Can you work these out from the model? Positions are in its coordinate system, mm. A direction names the side the tool comes from. Coordinates: 2 decimals unless noted, no trailing zeros. Order: outer loops, then holes, each group sorted by start corner. A loop starts at its lowest first (then second) coordinate and runs counter-clockwise, first axis right, second up.
```python
from build123d import *

# Parameters (mm, degrees)
F0_R     = 10
F1_DEPTH = 12


with BuildPart() as f1:
    # F0 (on Front) → F1 (new body)
    with BuildSketch(Plane.XZ):
        with BuildLine():
            Line((0, 20), (0, 0))
            Line((0, 0), (20, 0))
            Line((20, 0), (20, -10))
            Line((20, -10), (84, -10))
            Line((84, -10), (84, 0))
            Line((84, 0), (104, 0))
            Line((104, 0), (104, 20))
            ThreePointArc((104, 20), (92.284271, 48.284271), (64, 60))
            Line((64, 60), (40, 60))
            ThreePointArc((40, 60), (11.715729, 48.284271), (0, 20))
        make_face()
        with Locations((52, 40)):
            Circle(F0_R, mode=Mode.SUBTRACT)
    extrude(amount=F1_DEPTH)


solid = f1.part
```
1. Please list where these lines run through material, in increasing order: probe 1 along Z at (x, y) = (52, -3.25); probe 2 along Z at (x, y) = (59, -5); probe 3 along Z at (x, y) = (72, -9.5).
Completed:
probe 1: z = -10 to 30, 50 to 60
probe 2: z = -10 to 32.86, 47.14 to 60
probe 3: z = -10 to 59.19
2. Thinking about a two-plate mould opening in X: for faces 1 (the cylindrical face through (92.594, -5.916, 47.972)), 2 (the cylindrical face through (44, -6, 34)), 3 (the cylindrical face through (12.028, -5.916, 48.594)), 4 (the flat face through (51, -12, 25)), which applies, pulls with the +X half, pulls with the -X half, needs draft (parallel to the pull), parting line crosses it, or undercut?
Completed:
face 1: pulls with the +X half
face 2: undercut
face 3: pulls with the -X half
face 4: needs draft
3. Imagine slicing it at D-D on z = -4. Please give me the cut outline in (x, y), then the cut area to 3 significant figures.
Completed:
outline: (20, -12) - (84, -12) - (84, 0) - (20, 0) - close
area: 768 mm2
4. Imagine slicing it at B-B on y = -10.25. Please give me the cut outline in (x, z), then the cut area to 3 significant figures.
Completed:
outline: (0, 0) - (20, 0) - (20, -10) - (84, -10) - (84, 0) - (104, 0) - (104, 20) arc R40 ccw to (64, 60) - (40, 60) arc R40 ccw to (0, 20) - close; hole circle Ø20 at (52, 40)
area: 5,880 mm2
5. Imagine slicing it at A-A on x = 52. Please give me the cut outline in (y, z).
Completed:
outline: (-12, -10) - (0, -10) - (0, 30) - (-12, 30) - close; (-12, 50) - (0, 50) - (0, 60) - (-12, 60) - close
6. I'm going to push flat-ended pins straight in: pin 1 (8 mm diameter, centred on x = 43, z = 40.5, fed in from +Y); pin 2 (1.5 mm diameter, centred on x = 79.5, y = -3.5, fed in from +Z); pin 3 (5 mm diameter, centred on x = 18, y = -4, fed in from +Z); pin 4 (6 mm diameter, centred on y = -4.5, z = 46, fed in from +X). Where does each tip first touch, or does it pass through?
Completed:
pin 1: stops at y = 0
pin 2: stops at z = 57.18
pin 3: stops at z = 54.92
pin 4: stops at x = 96.73
7. On a 3-axis mill with a long thin cutter (end or side, diameter ignored), from which of +Z, -Z, +X, -X, +Y, -Y can I reach the whole of each face in a straight line? I mean faces 5 (the flat face through (84, -6, -5)), 6 (the flat face through (10, -6, 0)), 7 (the flat face through (52, -6, -10)). Say none if no direction works.
Completed:
face 5: -Z, +X, +Y, -Y
face 6: -Z, -X, +Y, -Y
face 7: -Z, +X, -X, +Y, -Y
8. Imagine slicing it at C-C on z = 40. Please give me the cut outline in (x, y).
Completed:
outline: (5.36, -12) - (42, -12) - (42, 0) - (5.36, 0) - close; (62, -12) - (98.64, -12) - (98.64, 0) - (62, 0) - close
